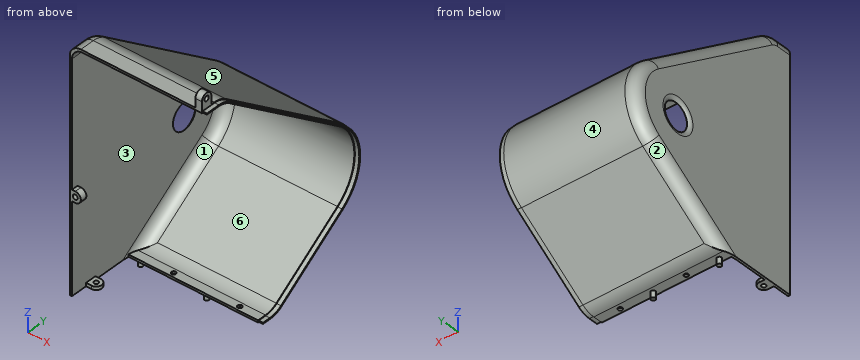
from build123d import *

# Parameters (mm, degrees)
CROQUIS1_R              = 12
SALIENTE_EXTRUIR1_DEPTH = 120
CORTAR_EXTRUIR1_DEPTH   = 118
REDONDEO1_R             = 20
CROQUIS3_W              = 250
CROQUIS3_H              = 250
CORTAR_EXTRUIR2_DEPTH   = 298.866030678
CROQUIS4_R              = 2
CORTAR_EXTRUIR3_DEPTH   = 20
CROQUIS5_R              = 2
SALIENTE_EXTRUIR2_DEPTH = 6
REDONDEO2_R             = 10
REDONDEO4_START         = 2.145107019
REDONDEO4_DEPTH         = 118.854892981
REDONDEO4_START_2       = 4.250447227
REDONDEO4_2_DEPTH       = 115.749552773
SALIENTE_EXTRUIR3_DEPTH = 4
CROQUIS7_R              = 2.25
SALIENTE_EXTRUIR4_DEPTH = 6
CROQUIS9_R              = 2.25
SALIENTE_EXTRUIR5_DEPTH = 6
CROQUIS10_R             = 2
SALIENTE_EXTRUIR6_DEPTH = 3
REDONDEO5_R             = 5


with BuildPart() as part:
    # Croquis1 → Saliente-Extruir1 (new body)
    with BuildSketch(Plane(origin=(0, 0, 0), x_dir=(0, 0, -1), z_dir=(1, 0, 0))):
        with BuildLine():
            Line((-200, 0), (200, 0))
            Line((200, 0), (200, 45))
            Line((200, 45), (175, 70))
            Line((175, 70), (17.023437057, 70))
            Line((17.023437057, 70), (17.023437057, 75))
            Line((17.023437057, 75), (-33.279638053, 146.01182459))
            ThreePointArc((-33.279638053, 146.01182459), (-69.531086216, 164.997556821), (-106.170314621, 146.771409007))
            Line((-106.170314621, 146.771409007), (-200, 20))
            Line((-200, 20), (-200, 0))
        make_face()
        with Locations((-70, 120)):
            Circle(CROQUIS1_R, mode=Mode.SUBTRACT)
    extrude(amount=SALIENTE_EXTRUIR1_DEPTH)

    # Croquis2 → Cortar-Extruir1 (cut)
    with BuildSketch(Plane(origin=(120, 0, 0), x_dir=(0, 0, -1), z_dir=(1, 0, 0))):
        with BuildLine():
            Line((35.023437057, 60), (35.023437057, 68))
            Line((35.023437057, 68), (174.171572875, 68))
            Line((174.171572875, 68), (198, 44.171572875))
            Line((198, 44.171572875), (198, 0))
            Line((198, 0), (-198, 0))
            Line((-198, 0), (-198, 19.340364538))
            Line((-198, 19.340364538), (-104.562745082, 145.581568607))
            ThreePointArc((-104.562745082, 145.581568607), (-69.551926829, 162.997665407), (-34.91165414, 144.855743497))
            Line((-34.91165414, 144.855743497), (15.023437057, 74.363394288))
            Line((15.023437057, 74.363394288), (15.023437057, 60))
            Line((15.023437057, 60), (35.023437057, 60))
        make_face()
    extrude(amount=-CORTAR_EXTRUIR1_DEPTH, mode=Mode.SUBTRACT)

    # Redondeo1
    redondeo1_edges = [part.edges().sort_by_distance(p)[0] for p in [
        (60, 20, 200),
        (60, 70, -175),
        (60, 45, -200),
        (61, 19.340364538, 198),
        (61, 68, -174.171572875),
        (61, 44.171572875, -198),
    ]]
    fillet(redondeo1_edges, radius=REDONDEO1_R)

    # Croquis3 → Cortar-Extruir2 (cut, through all)
    with BuildSketch(Plane(origin=(0, 0, -17.023437057), x_dir=(-1, 0, 0), z_dir=(0, 0, -1))):
        with Locations((-60, 64.142135624)):
            Rectangle(CROQUIS3_W, CROQUIS3_H)
    extrude(amount=CORTAR_EXTRUIR2_DEPTH, mode=Mode.SUBTRACT)

    # Croquis4 → Cortar-Extruir3 (cut)
    with BuildSketch(Plane(origin=(0, 0, -17.023437057), x_dir=(-1, 0, 0), z_dir=(0, 0, -1))):
        with Locations((-100, 64)):
            Circle(CROQUIS4_R)
        with Locations((-40, 64)):
            Circle(CROQUIS4_R)
    extrude(amount=-CORTAR_EXTRUIR3_DEPTH, mode=Mode.SUBTRACT)

    # Croquis5 → Saliente-Extruir2 (add)
    with BuildSketch(Plane(origin=(0, 0, -17.023437057), x_dir=(-1, 0, 0), z_dir=(0, 0, -1))):
        with Locations(Location((-70, 64, 0), (0, 0, 180))):
            Circle(CROQUIS5_R)
        with Locations(Location((-10, 64, 0), (0, 0, 180))):
            Circle(CROQUIS5_R)
    extrude(amount=SALIENTE_EXTRUIR2_DEPTH)

    # Redondeo2
    redondeo2_edges = [part.edges().sort_by_distance(p)[0] for p in [
        (0, 110.505912295, 8.128100498),
        (0, 6.701822688, 200),
        (0, 19.668072416, 198.993602972),
        (0, 86.036729193, 151.123005004),
        (0, 164.997556821, 69.531086216),
        (2, 6.372004957, 198),
        (2, 19.008436953, 196.993602972),
        (2, 109.609568893, 9.944108542),
        (2, 162.997665407, 69.551926829),
        (2, 85.111991262, 149.319220235),
    ]]
    fillet(redondeo2_edges, radius=REDONDEO2_R)

    # Redondeo4: read off the stored shape, not the designer's step
    # Redondeo4 outline → Redondeo4 (cut)
    with BuildSketch(Plane.YZ.offset(REDONDEO4_START)):
        with BuildLine():
            Line((75, -17.023437057), (80.194753812, -13.343597922))
            ThreePointArc((80.194753812, -13.343597922), (74.700110648, -16.081286061), (68.633942883, -17.023437057))
            Line((68.633942883, -17.023437057), (75, -17.023437057))
        make_face()
    extrude(amount=REDONDEO4_DEPTH, mode=Mode.SUBTRACT)

    # Redondeo4 2 outline → Redondeo4 2 (add)
    with BuildSketch(Plane.YZ.offset(REDONDEO4_START_2)):
        with BuildLine():
            Line((74.363394288, -15.023437057), (79.5581481, -11.343597922))
            ThreePointArc((79.5581481, -11.343597922), (74.063504936, -14.081286061), (67.997337171, -15.023437057))
            Line((67.997337171, -15.023437057), (74.363394288, -15.023437057))
        make_face()
    extrude(amount=REDONDEO4_2_DEPTH)

    # Croquis6 → Saliente-Extruir3 (add)
    with BuildSketch(Plane(origin=(120, 0, 0), x_dir=(0, 0, -1), z_dir=(1, 0, 0))):
        with BuildLine():
            Line((16.523437057, 60.5), (16.523437057, 68.633942883))
            ThreePointArc((16.523437057, 68.633942883), (15.604839835, 74.548456453), (12.9355939, 79.905733538))
            Line((12.9355939, 79.905733538), (-33.687642075, 145.722804317))
            ThreePointArc((-33.687642075, 145.722804317), (-69.536296369, 164.497583967), (-105.768422236, 146.473948907))
            Line((-105.768422236, 146.473948907), (-195.673803002, 25.00458928))
            ThreePointArc((-195.673803002, 25.00458928), (-198.518762898, 19.51146174), (-199.5, 13.403645376))
            Line((-199.5, 13.403645376), (-199.5, 0.5))
            Line((-199.5, 0.5), (-198.5, 0.5))
            Line((-198.5, 0.5), (-198.5, 12.744009914))
            ThreePointArc((-198.5, 12.744009914), (-197.468443047, 19.165047629), (-194.477587772, 24.939874017))
            Line((-194.477587772, 24.939874017), (-104.964637467, 145.879028707))
            ThreePointArc((-104.964637467, 145.879028707), (-69.546716676, 163.49763826), (-34.503650118, 145.144763771))
            Line((-34.503650118, 145.144763771), (11.751601944, 79.847168373))
            ThreePointArc((11.751601944, 79.847168373), (14.557732286, 74.21515913), (15.523437057, 67.997337171))
            Line((15.523437057, 67.997337171), (15.523437057, 60.5))
            Line((15.523437057, 60.5), (16.523437057, 60.5))
        make_face()
    extrude(amount=SALIENTE_EXTRUIR3_DEPTH)

    # Croquis7 → Saliente-Extruir4 (add)
    with BuildSketch(Plane.XZ):
        with BuildLine():
            Line((2, 75), (5, 75))
            ThreePointArc((5, 75), (10, 70), (5, 65))
            Line((5, 65), (2, 65))
            Line((2, 65), (2, 75))
        make_face()
        with Locations(Location((5, 70, 0), (0, 0, 270))):
            Circle(CROQUIS7_R, mode=Mode.SUBTRACT)
    extrude(amount=-SALIENTE_EXTRUIR4_DEPTH)

    # Croquis9 → Saliente-Extruir5 (add)
    with BuildSketch(Plane(origin=(120, 0, 0), x_dir=(0, 0, -1), z_dir=(1, 0, 0))):
        with BuildLine():
            Line((-200, 0), (-208, 0))
            ThreePointArc((-208, 0), (-213, 5), (-208, 10))
            Line((-208, 10), (-200, 10))
            Line((-200, 10), (-200, 0))
        make_face()
        with Locations((-208, 5)):
            Circle(CROQUIS9_R, mode=Mode.SUBTRACT)
    extrude(amount=-SALIENTE_EXTRUIR5_DEPTH)

    # Croquis10 → Saliente-Extruir6 (add)
    with BuildSketch(Plane(origin=(0, 0, -17.023437057), x_dir=(-1, 0, 0), z_dir=(0, 0, -1))):
        with BuildLine():
            Line((-2, 15), (-7, 15))
            ThreePointArc((-7, 15), (-12, 20), (-7, 25))
            Line((-7, 25), (-2, 25))
            Line((-2, 25), (-2, 15))
        make_face()
        with Locations((-7, 20)):
            Circle(CROQUIS10_R, mode=Mode.SUBTRACT)
    extrude(amount=-SALIENTE_EXTRUIR6_DEPTH)

    # Redondeo5
    # the kernel refuses this fillet: 5 mm, written as the material it takes off along each edge
    with BuildSketch(Plane(origin=(0, 120, 70), x_dir=(0, 0, -1), z_dir=(0, -1, 0))) as redondeo5_piece_1:
        with BuildLine():
            CenterArc((16, 5), REDONDEO5_R, 216.869897646, 53.130102354)
            Line((12, 2), (11.92, 1.94))
            ThreePointArc((11.92, 1.94), (11.9, 1), (11.9, 0))
            Line((11.9, 0), (12, -0.1))
            Line((12, -0.1), (16, -0.1))
            Line((16, -0.1), (16, 0))
        make_face()
    revolve(axis=Axis((0, 120, 70), (1, 0, 0)), mode=Mode.SUBTRACT)


solid = part.part
Check sheet for the modelled part. Datum: model origin and axes. Units: mm. Face numbers are marked on the shaded views. A direction names the side the tool comes from. Give positions to 0.01 mm unless a question says otherwise; leave off trailing zeros. Loops run counter-clockwise (first coordinate to the right, second up) from the corner with the lowest first, then second, coordinate; pieces in that order, holes last. Notation, with made-up numbers: M -18,89.25 L 21,89.25 A5 cw 21,98.25 Z; hole C 32,7.5 d4. An arc over 180 degrees is marked long. Answer as a JSON object with one key per item and string values. Group by question number.
Q1. Cross-section at A-A on x = 47.5. Record the cut outline in (y, z).
Q2. Release check for a two-part mould opening along Z. For the marked faces 1, 2, 3 and 4 record: released by +Z, released by -Z, zero draft, split by the parting line, or undercut.
Q3. Access from +Z, -Z, +X, -X, +Y, -Y to the whole of each face (thin tool, end or side, straight path). Record for the marked faces 5 and 6.
Q4. Go/stop test with flat-tipped pins: P1, Ø3.5, axis at x = 3, y = 2.5, coming from the +Z side; P2, Ø9, axis at x = 84, y = 65.5, coming from the +Z side; P3, Ø3, axis at x = 121, y = 7.5, coming from the -Z side. Record where each tip stops, or that it passes through.
Q5. Material ranges on line 1 along X through (y, z) = (2, 70); line 2 along X through (y, z) = (74, 35.5); line 3 along Z through (x, y) = (23.5, 97), recorded low to high. Write a range as [from, to].
Evaluation:
{
 "1": {"outline": "M 0,198 L 12.74,198 A20 cw 24.64,194.08 L 145.58,104.56 A43 cw 144.86,34.91 L 79.56,-11.34 A20 cw 68,-15.02 L 60,-15.02 L 60,-17.02 L 68.63,-17.02 A20 ccw 80.19,-13.34 L 146.01,33.28 A45 ccw 146.77,106.17 L 25.3,196.08 A20 ccw 13.4,200 L 0,200 Z"},
 "2": {"face 1": "undercut", "face 2": "released by -Z", "face 3": "undercut", "face 4": "split by the parting line"},
 "3": {"face 5": "+Z, +X, -X, +Y", "face 6": "+X, -Y"},
 "4": {"P1": "stops at z = 198.51", "P2": "stops at z = 169.65", "P3": "stops at z = 198"},
 "5": {"line 1": "x = [0, 2.75], [7.25, 10]", "line 2": "x = [0, 2]", "line 3": "z = [-1.44, 1.01], [140.52, 143.01]"}
}
